Input: part model. Units: mm. Frame: model coordinates. A direction names the side the tool comes from. Coordinates: 2 decimals unless noted, no trailing zeros. Loops run counter-clockwise (first coordinate to the right, second up) from the corner with the lowest first, then second, coordinate; pieces in that order, holes last.
(1) Contact query for a flat-ended pin moving along its axis: P1, Ø2.5, axis at x = -44.5, z = 0, coming from the -Y side. Output: stop coordinate, or through.
(2) Section D-D, the plane z = -34. Return loops of the section in (x, y), then the cut area to 3 significant figures.
(3) Mould query, pull axis X, two halves, no side actions, for faces 1 (the face through (-1, 0, -1)), 2 (the face through (-43.32, 1.48, -1.08)), 3 (the face through (65, 1, 1)). Classes: released by +X, released by -X, zero draft, split by the parting line, or undercut.
(4) Line query: L1, parallel to X at y = 1.9, z = 4; L2, parallel to Z at x = 44.5, y = 1.55; L3, parallel to Z at x = 23, y = 0.65. Output: solid intervals per line, ascending.
(5) Section B-B, the plane y = 1.55. Return loops of the section in (x, z).
(6) Section A-A, the plane z = 0. Return loops of the section in (x, y), then the cut area to 3 significant figures.
(7) Section C-C, the plane x = -44.5. Return loops of the section in (y, z).
(8) Set-up query: faces 4 (the face through (-1, 1, -60)), 5 (the face through (-16, 1, 44.5)). Return all of +Z, -Z, +X, -X, +Y, -Y with unobstructed straight access to the full face (end or side cutting, diameter ignored); none if empty.
```python
from build123d import *

# Parameters (mm, degrees)
SKETCH1_W           = 130
SKETCH1_H           = 120
BOSS_EXTRUDE1_DEPTH = 3
CUT_EXTRUDE1_START  = -4
SKETCH2_W           = 20
SKETCH2_H           = 89
CUT_EXTRUDE1_DEPTH  = 5
CUT_EXTRUDE2_START  = -4
SKETCH3_R           = 1.6
CUT_EXTRUDE2_DEPTH  = 5


with BuildPart() as part:
    # Sketch1 → Boss-Extrude1 (new body)
    with BuildSketch(Plane(origin=(0, 0, 0), x_dir=(1, 0, 0), z_dir=(0, 1, 0))):
        Rectangle(SKETCH1_W, SKETCH1_H)
    extrude(amount=BOSS_EXTRUDE1_DEPTH)

    # Sketch2 → Cut-Extrude1 (cut)
    with BuildSketch(Plane(origin=(0, 3, 0), x_dir=(1, 0, 0), z_dir=(0, 1, 0)).offset(CUT_EXTRUDE1_START)):
        with Locations((-16.25, 0)):
            Rectangle(SKETCH2_W, SKETCH2_H)
    cut_extrude1 = extrude(amount=CUT_EXTRUDE1_DEPTH, mode=Mode.SUBTRACT)

    # Mirror1: Cut-Extrude1 across plane
    add(cut_extrude1.mirror(Plane(origin=(0, 0, 0), x_dir=(0, 0, 1), z_dir=(1, 0, 0))), mode=Mode.SUBTRACT)

    # Sketch3 → Cut-Extrude2 (cut)
    with BuildSketch(Plane(origin=(0, 3, 0), x_dir=(1, 0, 0), z_dir=(0, 1, 0)).offset(CUT_EXTRUDE2_START)):
        with Locations((44.5, 0)):
            Circle(SKETCH3_R)
    cut_extrude2 = extrude(amount=CUT_EXTRUDE2_DEPTH, mode=Mode.SUBTRACT)

    # Mirror2: Cut-Extrude2 across plane
    add(cut_extrude2.mirror(Plane(origin=(0, 0, 0), x_dir=(0, 0, 1), z_dir=(1, 0, 0))), mode=Mode.SUBTRACT)


solid = part.part
```
Report:
1. P1: passes through
2. outline: (-65, 0) - (-26.25, 0) - (-26.25, 3) - (-65, 3) - close; (-6.25, 0) - (6.25, 0) - (6.25, 3) - (-6.25, 3) - close; (26.25, 0) - (65, 0) - (65, 3) - (26.25, 3) - close
2. area: 270 mm2
3. face 1: zero draft
3. face 2: undercut
3. face 3: released by +X
4. L1: x = -65 to -26.25, -6.25 to 6.25, 26.25 to 65
4. L2: z = -60 to -1.6, 1.6 to 60
4. L3: z = -60 to -44.5, 44.5 to 60
5. outline: (-65, -60) - (65, -60) - (65, 60) - (-65, 60) - close; hole circle Ø3.2 at (-44.5, 0); hole (-26.25, -44.5) - (-6.25, -44.5) - (-6.25, 44.5) - (-26.25, 44.5) - close; hole (6.25, -44.5) - (26.25, -44.5) - (26.25, 44.5) - (6.25, 44.5) - close; hole circle Ø3.2 at (44.5, 0)
6. outline: (-65, 0) - (-46.1, 0) - (-46.1, 3) - (-65, 3) - close; (-42.9, 0) - (-26.25, 0) - (-26.25, 3) - (-42.9, 3) - close; (-6.25, 0) - (6.25, 0) - (6.25, 3) - (-6.25, 3) - close; (26.25, 0) - (42.9, 0) - (42.9, 3) - (26.25, 3) - close; (46.1, 0) - (65, 0) - (65, 3) - (46.1, 3) - close
6. area: 251 mm2
7. outline: (0, -60) - (3, -60) - (3, -1.6) - (0, -1.6) - close; (0, 1.6) - (3, 1.6) - (3, 60) - (0, 60) - close
8. face 4: -Z, +X, -X, +Y, -Y
8. face 5: +Y, -Y
